Source: three-view drawing plus pictorial views. Frame: mm from the lowest corner of the part. A direction names the side the tool comes from. Give positions to 0.01 mm unless a question says otherwise; leave off trailing zeros. Order: outer loops, then holes, each group sorted by start corner. A loop starts at its lowest first (then second) coordinate and runs counter-clockwise, first axis right, second up. Notation, with made-up numbers: (72.5, 75) -> (112.5, 75) arc R27 cw to (112.5, 111) -> close; hole circle Ø7 at (25.5, -30.75). An arc over 180 degrees is marked (long way). Answer in a Markdown table with one row per item. Add a question column.
Q1. Cut plane A-A on y = 25. Return the cut outline in (x, z).
Q2. Set-up query: the marked faces 4 and 5. Return all of +Z, -Z, +X, -X, +Y, -Y with unobstructed straight access to the full face (end or side cutting, diameter ignored); none if empty.
Q3. Pull-direction query (X, two-part tool) for the marked faces 1, 2 and 3; classes: +X half, -X half, draft (parallel to the pull), parting line (faces both ways), or undercut.
Q4. Contact query for flat-ended pins moving along their axis: P1, Ø16, axis at x = 25, y = 25, coming from the +Z side; P2, Ø2, axis at y = 40.5, z = 0.5, coming from the -X side (1 decimal); P3, Ø2.5, axis at y = 37, z = 2, coming from the -X side; P4, Ø1.5, axis at x = 13.5, z = 2.5, coming from the +Y side. Output: stop coordinate, or through.
Q5. Line query: line 1 along Y through (x, z) = (25, 1.25); line 2 along X through (y, z) = (35.5, 0.25); line 3 along X through (y, z) = (41, 4). Output: solid intervals per line, ascending. Write a range as from..to.
Q6. Cut plane C-C on z = 0.85. Return the cut outline in (x, y), and give its area (3 significant figures).
Q7. Cut plane B-B on x = 15.5. Count the separate pieces of the cut face and the enclosed holes in it, and give its area (3 significant figures).
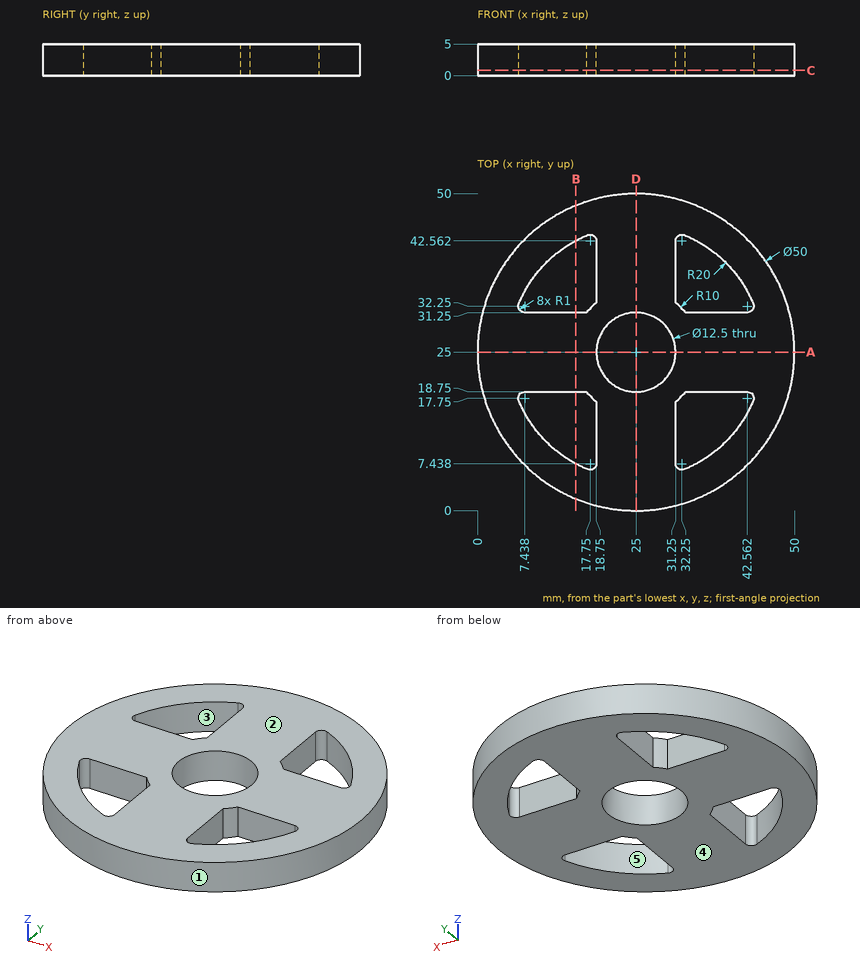
Completed:
| question | item | result |
|---|---|---|
| 1 | outline | (0, 0) -> (18.75, 0) -> (18.75, 5) -> (0, 5) -> close; (31.25, 0) -> (50, 0) -> (50, 5) -> (31.25, 5) -> close |
| 2 | face 4 | -Z, +X, -X, +Y, -Y |
| 2 | face 5 | +Z, -Z |
| 3 | face 1 | parting line |
| 3 | face 2 | draft |
| 3 | face 3 | undercut |
| 4 | P1 | stops at z = 5 |
| 4 | P2 | stops at x = 4.6 |
| 4 | P3 | stops at x = 2.43 |
| 4 | P4 | stops at y = 47.57 |
| 5 | line 1 | y = 0..18.75, 31.25..50 |
| 5 | line 2 | x = 2.31..7.98, 18.75..31.25, 42.02..47.69 |
| 5 | line 3 | x = 5.79..13, 18.75..31.25, 37..44.21 |
| 6 | outline | circle Ø50 at (25, 25); hole (6.51, 17.37) arc R20 ccw to (17.37, 6.51) arc R1 ccw to (18.75, 7.44) -> (18.75, 17.19) arc R10 cw to (17.19, 18.75) -> (7.44, 18.75) arc R1 ccw to start; hole (6.51, 32.63) arc R1 ccw to (7.44, 31.25) -> (17.19, 31.25) arc R10 cw to (18.75, 32.81) -> (18.75, 42.56) arc R1 ccw to (17.37, 43.49) arc R20 ccw to start; hole circle Ø12.5 at (25, 25); hole (31.25, 7.44) arc R1 ccw to (32.63, 6.51) arc R20 ccw to (43.49, 17.37) arc R1 ccw to (42.56, 18.75) -> (32.81, 18.75) arc R10 cw to (31.25, 17.19) -> close; hole (31.25, 32.81) arc R10 cw to (32.81, 31.25) -> (42.56, 31.25) arc R1 ccw to (43.49, 32.63) arc R20 ccw to (32.63, 43.49) arc R1 ccw to (31.25, 42.56) -> close |
| 6 | area | 1,420 mm² |
| 7 | separate pieces | 3 |
| 7 | enclosed holes | 0 |
| 7 | area | 118 mm² |
